```python
from build123d import *
from build123d.topology import SkipClean

# Parameters (mm, degrees)
SKETCH1_R                            = 30
BOSS_EXTRUDE1_DEPTH                  = 4
BOSS_EXTRUDE2_REACH                  = 44.615
BOSS_EXTRUDE2_END_RADIUS             = 30
BOSS_EXTRUDE2_DIRECTION_2_REACH      = 44.615
BOSS_EXTRUDE2_DIRECTION_2_END_RADIUS = 30
SKETCH3_OUTSIDE_W                    = 78.092
SKETCH3_OUTSIDE_H                    = 69.092
SKETCH3_OUTSIDE_R                    = 21.5
CUT_EXTRUDE2_DEPTH                   = 12.5
BOSS_EXTRUDE3_DEPTH                  = 18
BOSS_EXTRUDE4_DEPTH                  = 15
BOSS_EXTRUDE5_DEPTH                  = 15
CUT_EXTRUDE3_DEPTH                   = 44.292609069
CUT_EXTRUDE3_DEPTH_BACK              = 44.292609069
SKETCH8_R                            = 2
CUT_EXTRUDE8_DEPTH                   = 48.077064479
CUT_EXTRUDE8_DEPTH_BACK              = 48.077064479
CUT_EXTRUDE9_DEPTH                   = 59.659818207
CUT_EXTRUDE11_DEPTH                  = 20
CUT_EXTRUDE12_DEPTH                  = 20
CUT_EXTRUDE13_DEPTH                  = 20
CUT_EXTRUDE14_DEPTH                  = 44.292609069
CUT_EXTRUDE14_DEPTH_BACK             = 44.292609069
SKETCH25_W                           = 66.075437062
SKETCH25_H                           = 20.142243048
SKETCH26_R                           = 5
CUT_EXTRUDE15_DEPTH                  = 24
SKETCH27_R                           = 1.5
CUT_EXTRUDE16_DEPTH                  = 30
SKETCH28_R                           = 5
CUT_EXTRUDE17_DEPTH                  = 3
CUT_EXTRUDE18_DEPTH                  = 43.690748412
CUT_EXTRUDE18_DEPTH_BACK             = 43.690748412
SKETCH29_W                           = 43.412566799
SKETCH29_H                           = 13.326200919
SKETCH32_W                           = 50
SKETCH32_H                           = 12
BOSS_EXTRUDE6_DEPTH                  = 18
SKETCH35_W                           = 14
SKETCH35_H                           = 15
BOSS_EXTRUDE7_DEPTH                  = 9
CUT_EXTRUDE19_DEPTH                  = 49.746794766
CUT_EXTRUDE19_DEPTH_BACK             = 49.746794766
SKETCH37_R                           = 2
SKETCH36_R                           = 2
CUT_EXTRUDE20_DEPTH                  = 15
SKETCH39_W                           = 14
SKETCH39_H                           = 15
BOSS_EXTRUDE8_DEPTH                  = 9
SKETCH40_R                           = 2
CUT_EXTRUDE21_DEPTH                  = 10
CUT_EXTRUDE22_START                  = -9
SKETCH41_R                           = 5
CUT_EXTRUDE22_DEPTH                  = 9
CUT_EXTRUDE23_START                  = -9
SKETCH42_R                           = 5
CUT_EXTRUDE23_DEPTH                  = 9
FILLET1_R                            = 3
CUT_EXTRUDE24_START                  = -19
CUT_EXTRUDE24_OUTLINE_R              = 1.5
CUT_EXTRUDE24_DEPTH                  = 19
CUT_EXTRUDE24_START_2                = -7
CUT_EXTRUDE24_2_DEPTH                = 14


with BuildPart() as part:
    # Sketch1 → Boss-Extrude1 (new body)
    with BuildSketch(Plane(origin=(0, 0, 0), x_dir=(1, 0, 0), z_dir=(0, 1, 0))):
        with Locations(Location((0, 0, 0), (0, 0, 270))):
            Circle(SKETCH1_R)
    extrude(amount=BOSS_EXTRUDE1_DEPTH)

    # Boss-Extrude2: up to this cylinder (the profile starts inside it)
    with SkipClean():  # the faces are left unmerged after this step: merging them gives an invalid solid
        boss_extrude2_end = Plane(origin=(0, 9.396175, 0), z_dir=(0, -1, 0)) * Cylinder(BOSS_EXTRUDE2_END_RADIUS, 150.23, mode=Mode.PRIVATE)
        # Sketch2 → Boss-Extrude2 (add, up to the surface)
        with BuildSketch(Plane(origin=(0, 0, 0), x_dir=(0, 0, -1), z_dir=(1, 0, 0)), mode=Mode.PRIVATE) as boss_extrude2_sk1:
            Polygon((0, 4), (21.5, 4), (9, 16.5), (-9, 16.5), (-21.5, 4), align=None)
        boss_extrude2_tool1 = extrude(boss_extrude2_sk1.sketch, amount=BOSS_EXTRUDE2_REACH, mode=Mode.PRIVATE) & boss_extrude2_end
        add(boss_extrude2_tool1.solids().sort_by_distance((0, 9.396175, 0))[0])

    # Boss-Extrude2 direction 2: up to this cylinder (the profile starts inside it)
    with SkipClean():  # the faces are left unmerged after this step: merging them gives an invalid solid
        boss_extrude2_direction_2_end = Plane(origin=(0, 9.396175, 0), z_dir=(0, -1, 0)) * Cylinder(BOSS_EXTRUDE2_DIRECTION_2_END_RADIUS, 150.23, mode=Mode.PRIVATE)
        # Sketch2 → Boss-Extrude2 direction 2 (add, up to the surface)
        with BuildSketch(Plane(origin=(0, 0, 0), x_dir=(0, 0, -1), z_dir=(1, 0, 0)), mode=Mode.PRIVATE) as boss_extrude2_direction_2_sk1:
            Polygon((0, 4), (21.5, 4), (9, 16.5), (-9, 16.5), (-21.5, 4), align=None)
        boss_extrude2_direction_2_tool1 = extrude(boss_extrude2_direction_2_sk1.sketch, amount=-BOSS_EXTRUDE2_DIRECTION_2_REACH, mode=Mode.PRIVATE) & boss_extrude2_direction_2_end
        add(boss_extrude2_direction_2_tool1.solids().sort_by_distance((0, 9.396175, 0))[0])

    # SurfaceCut1
    split(bisect_by=Plane(origin=(0, 12.75, -12.75), x_dir=(1, 0, 0), z_dir=(0, 0.7071067811865558, -0.7071067811865392)), keep=Keep.BOTTOM)

    # SurfaceCut2
    split(bisect_by=Plane(origin=(0, 12.75, 12.75), x_dir=(1, 0, 0), z_dir=(0, 0.7071067811865509, 0.7071067811865442)), keep=Keep.BOTTOM)

    # Sketch3 outside → Cut-Extrude2 (cut)
    with BuildSketch(Plane(origin=(0, 4, 0), x_dir=(1, 0, 0), z_dir=(0, 1, 0))):
        Rectangle(SKETCH3_OUTSIDE_W, SKETCH3_OUTSIDE_H)
        Circle(SKETCH3_OUTSIDE_R, mode=Mode.SUBTRACT)
    extrude(amount=CUT_EXTRUDE2_DEPTH, mode=Mode.SUBTRACT)

    # Sketch5 → Boss-Extrude3 (add)
    with BuildSketch(Plane(origin=(0, 0, 0), x_dir=(-1, 0, 0), z_dir=(0, -1, 0))):
        Polygon((0, -6), (-17.5, -6), (-17.5, 6), (17.5, 6), (17.5, -6), align=None)
    extrude(amount=BOSS_EXTRUDE3_DEPTH)

    # Sketch6 → Boss-Extrude4 (add)
    with BuildSketch(Plane.XZ):
        Polygon((0, 15), (7, 15), (7, 6), (-7, 6), (-7, 15), align=None)
    extrude(amount=BOSS_EXTRUDE4_DEPTH)

    # Sketch7 → Boss-Extrude5 (add)
    with BuildSketch(Plane.XZ):
        Polygon((0, -15), (7, -15), (7, -6), (-7, -6), (-7, -15), align=None)
    extrude(amount=BOSS_EXTRUDE5_DEPTH)

    # Sketch8 → Cut-Extrude3 (cut, two sides: drawn at the far end of the back side and taken through both)
    with BuildSketch(Plane.XY.offset(-CUT_EXTRUDE3_DEPTH_BACK)):
        with Locations((-12.5, -12.5)):
            Circle(SKETCH8_R)
        with Locations((12.5, -12.5)):
            Circle(SKETCH8_R)
    extrude(amount=CUT_EXTRUDE3_DEPTH + CUT_EXTRUDE3_DEPTH_BACK, mode=Mode.SUBTRACT)

    # Sketch16 → Cut-Extrude8 (cut, two sides: drawn at the far end of the back side and taken through both)
    with BuildSketch(Plane.XY.offset(6).offset(-CUT_EXTRUDE8_DEPTH_BACK)):
        Polygon((17.5, -18), (17.5, -14.5), (14, -18), align=None)
        Polygon((-17.5, -18), (-14, -18), (-17.5, -14.5), align=None)
    extrude(amount=CUT_EXTRUDE8_DEPTH + CUT_EXTRUDE8_DEPTH_BACK, mode=Mode.SUBTRACT)

    # Sketch17 → Cut-Extrude9 (cut, through all)
    with BuildSketch(Plane(origin=(10.365975269, -9.674910251, -8.062425209), x_dir=(-0.3613483622370374, 0.337258471421235, -0.8693009171531012), z_dir=(0.6355070151731325, -0.5931398808282571, -0.49428323402354774))):
        Polygon((-2.372510104, -6.189601271), (7.980636686, -0.706686759), (7.980636686, -10.965829024), align=None)
    extrude(amount=CUT_EXTRUDE9_DEPTH, mode=Mode.SUBTRACT)

    # Sketch19 → Cut-Extrude11 (cut)
    with BuildSketch(Plane(origin=(-10.365975269, -9.674910251, -8.062425209), x_dir=(0.3613483622370374, 0.33725847142123494, -0.8693009171531012), z_dir=(0.6355070151731324, 0.5931398808282571, 0.4942832340235476))):
        Polygon((-2.372510104, -6.189601271), (7.980636686, -10.965829024), (7.980636686, -0.706686759), align=None)
    extrude(amount=-CUT_EXTRUDE11_DEPTH, mode=Mode.SUBTRACT)

    # Sketch20 → Cut-Extrude12 (cut)
    with BuildSketch(Plane(origin=(-10.365975269, -9.674910251, 8.062425209), x_dir=(-0.3613483622370374, -0.3372584714212349, -0.8693009171531013), z_dir=(0.6355070151731326, 0.593139880828257, -0.49428323402354757))):
        Polygon((2.372510104, -6.189601271), (-7.980636686, -0.706686759), (-7.980636686, -10.965829024), align=None)
    extrude(amount=-CUT_EXTRUDE12_DEPTH, mode=Mode.SUBTRACT)

    # Sketch21 → Cut-Extrude13 (cut)
    with BuildSketch(Plane(origin=(10.365975269, -9.674910251, 8.062425209), x_dir=(-0.3613483622370374, 0.3372584714212349, 0.8693009171531013), z_dir=(-0.6355070151731326, 0.593139880828257, -0.49428323402354757))):
        Polygon((-2.372510104, -6.189601271), (7.980636686, -0.706686759), (7.980636686, -10.965829024), align=None)
    extrude(amount=-CUT_EXTRUDE13_DEPTH, mode=Mode.SUBTRACT)

    # Sketch25 → Cut-Extrude14 (cut, two sides: drawn at the far end of the back side and taken through both)
    with BuildSketch(Plane.XY.offset(-CUT_EXTRUDE14_DEPTH_BACK)):
        with Locations((0, -10.071121524)):
            Rectangle(SKETCH25_W, SKETCH25_H)
    extrude(amount=CUT_EXTRUDE14_DEPTH + CUT_EXTRUDE14_DEPTH_BACK, mode=Mode.SUBTRACT)

    # Sketch26 → Cut-Extrude15 (cut)
    with BuildSketch(Plane(origin=(0, 16.5, 0), x_dir=(1, 0, 0), z_dir=(0, 1, 0))):
        with Locations(Location((-8, 0, 0), (0, 0, 270))):
            Circle(SKETCH26_R)
        with Locations(Location((8, 0, 0), (0, 0, 270))):
            Circle(SKETCH26_R)
    extrude(amount=-CUT_EXTRUDE15_DEPTH, mode=Mode.SUBTRACT)

    # Sketch27 → Cut-Extrude16 (cut)
    with BuildSketch(Plane(origin=(0, 16.5, 0), x_dir=(1, 0, 0), z_dir=(0, 1, 0))):
        with Locations(Location((0, 0, 0), (0, 0, 270))):
            Circle(SKETCH27_R)
    extrude(amount=-CUT_EXTRUDE16_DEPTH, mode=Mode.SUBTRACT)

    # Sketch28 → Cut-Extrude17 (cut)
    with BuildSketch(Plane.XZ):
        with Locations(Location((0, -15, 0), (0, 0, 270))):
            Circle(SKETCH28_R)
        with Locations(Location((22, 0, 0), (0, 0, 270))):
            Circle(SKETCH28_R)
        with Locations(Location((0, 15, 0), (0, 0, 270))):
            Circle(SKETCH28_R)
        with Locations(Location((-22, 0, 0), (0, 0, 270))):
            Circle(SKETCH28_R)
        with Locations(Location((-14, 12, 0), (0, 0, 270))):
            Circle(SKETCH28_R)
        with Locations(Location((14, 12, 0), (0, 0, 270))):
            Circle(SKETCH28_R)
        with Locations(Location((14, -12, 0), (0, 0, 270))):
            Circle(SKETCH28_R)
        with Locations(Location((-14, -12, 0), (0, 0, 270))):
            Circle(SKETCH28_R)
    extrude(amount=-CUT_EXTRUDE17_DEPTH, mode=Mode.SUBTRACT)

    # Sketch29 → Cut-Extrude18 (cut, two sides: drawn at the far end of the back side and taken through both)
    with BuildSketch(Plane(origin=(0, 0, 0), x_dir=(0, 0, -1), z_dir=(1, 0, 0)).offset(-CUT_EXTRUDE18_DEPTH_BACK)):
        with Locations((0.2062834, 10.66310046)):
            Rectangle(SKETCH29_W, SKETCH29_H)
    extrude(amount=CUT_EXTRUDE18_DEPTH + CUT_EXTRUDE18_DEPTH_BACK, mode=Mode.SUBTRACT)

    # Sketch32 → Boss-Extrude6 (add)
    with BuildSketch(Plane(origin=(0, 4, 0), x_dir=(1, 0, 0), z_dir=(0, 1, 0))):
        Rectangle(SKETCH32_W, SKETCH32_H)
    extrude(amount=BOSS_EXTRUDE6_DEPTH)

    # Sketch35 → Boss-Extrude7 (add)
    with BuildSketch(Plane(origin=(0, 0, -6), x_dir=(-1, 0, 0), z_dir=(0, 0, -1))):
        with Locations((0, 11.5)):
            Rectangle(SKETCH35_W, SKETCH35_H)
    extrude(amount=BOSS_EXTRUDE7_DEPTH)

    # Sketch37 → Cut-Extrude19 (cut, two sides: drawn at the far end of the back side and taken through both)
    with BuildSketch(Plane(origin=(0, 0, -6), x_dir=(-1, 0, 0), z_dir=(0, 0, -1)).offset(-CUT_EXTRUDE19_DEPTH_BACK)):
        with Locations((-12.5, 16.5)):
            Circle(SKETCH37_R)
        with Locations((12.5, 16.5)):
            Circle(SKETCH37_R)
    extrude(amount=CUT_EXTRUDE19_DEPTH + CUT_EXTRUDE19_DEPTH_BACK, mode=Mode.SUBTRACT)

    # Sketch36 → Cut-Extrude20 (cut)
    with BuildSketch(Plane(origin=(0, 19, 0), x_dir=(1, 0, 0), z_dir=(0, 1, 0))):
        with Locations(Location((0, 10, 0), (0, 0, 270))):
            Circle(SKETCH36_R)
    extrude(amount=-CUT_EXTRUDE20_DEPTH, mode=Mode.SUBTRACT)

    # Sketch39 → Boss-Extrude8 (add)
    with BuildSketch(Plane.XY.offset(6)):
        with Locations((0, 11.5)):
            Rectangle(SKETCH39_W, SKETCH39_H)
    extrude(amount=BOSS_EXTRUDE8_DEPTH)

    # Sketch40 → Cut-Extrude21 (cut)
    with BuildSketch(Plane(origin=(0, 19, 0), x_dir=(1, 0, 0), z_dir=(0, 1, 0))):
        with Locations(Location((0, -10, 0), (0, 0, 270))):
            Circle(SKETCH40_R)
    extrude(amount=-CUT_EXTRUDE21_DEPTH, mode=Mode.SUBTRACT)

    # Sketch41 → Cut-Extrude22 (cut)
    with BuildSketch(Plane.XZ.offset(-4).offset(CUT_EXTRUDE22_START)):
        with Locations(Location((-8, 0, 0), (0, 0, 90))):
            Circle(SKETCH41_R)
    extrude(amount=CUT_EXTRUDE22_DEPTH, mode=Mode.SUBTRACT)

    # Sketch42 → Cut-Extrude23 (cut)
    with BuildSketch(Plane.XZ.offset(-4).offset(CUT_EXTRUDE23_START)):
        with Locations(Location((8, 0, 0), (0, 0, 90))):
            Circle(SKETCH42_R)
    extrude(amount=CUT_EXTRUDE23_DEPTH, mode=Mode.SUBTRACT)

    # Fillet1
    fillet1_edges = [part.edges().sort_by_distance(p)[0] for p in [
        (25, 22, 0),
    ]]
    fillet(fillet1_edges, radius=FILLET1_R)

    # Cut-Extrude24: read off the stored shape, not the designer's step
    # Cut-Extrude24 outline → Cut-Extrude24 (cut)
    with BuildSketch(Plane.XZ.offset(-4).offset(CUT_EXTRUDE24_START)):
        Circle(CUT_EXTRUDE24_OUTLINE_R)
    extrude(amount=CUT_EXTRUDE24_DEPTH, mode=Mode.SUBTRACT)

    # Cut-Extrude24 2 outline → Cut-Extrude24 2 (cut)
    with BuildSketch(Plane.XY.offset(CUT_EXTRUDE24_START_2)):
        with BuildLine():
            Line((-25, 22), (-25, 19))
            ThreePointArc((-25, 19), (-24.121320344, 21.121320344), (-22, 22))
            Line((-22, 22), (-25, 22))
        make_face()
    extrude(amount=CUT_EXTRUDE24_2_DEPTH, mode=Mode.SUBTRACT)


solid = part.part
```
CAD build for the part. Positions are in the model's coordinates, mm. A direction names the side the tool comes from. Coordinates: 2 decimals unless noted, no trailing zeros. Order: outer loops, then holes, each group sorted by start corner. A loop starts at its lowest first (then second) coordinate and runs counter-clockwise, first axis right, second up.
(1) Saw through at B-B, the plane y = 1.5. Count the separate pieces of the cut face and the enclosed holes in it, and give its area (3 significant figures).
Solution:
separate pieces: 1
enclosed holes: 11
area: 1,740 mm2
(2) Which spindle directions (+Z, -Z, +X, -X, +Y, -Y) get a long thin tool onto all of the face, cutting with end or side? Do faces 5 (the face through (-2, 19, 11)), 6 (the face through (14, 3, -12)), 7 (the face through (0, 4, -10)), 8 (the face through (7, 11, -10)). Say none if no direction does.
Solution:
face 5: +Z, +X, -X, +Y
face 6: -Y
face 7: +Y
face 8: -Z, +X, +Y
(3) Pin check, flat tips, straight feed: pin 1 Ø7 at (x, y) = (0.5, 11.5) entering from -Z; pin 2 Ø1 at (x, y) = (17.5, 4) entering from +Z; pin 3 Ø2 at (y, z) = (12, -0.5) entering from -X. Stop position of each tip, or through.
Solution:
pin 1: stops at z = -15
pin 2: stops at z = 22
pin 3: stops at x = -25
(4) Saw through at A-A, the plane y = 16.5. Write the cut outline in (x, z), and give its area (3 significant figures).
Solution:
outline: (-25, -6) - (-14.5, -6) - (-14.5, 6) - (-25, 6) - close; (-10.5, -6) - (-7, -6) - (-7, -15) - (7, -15) - (7, -6) - (10.5, -6) - (10.5, 6) - (7, 6) - (7, 15) - (-7, 15) - (-7, 6) - (-10.5, 6) - close; (14.5, -6) - (25, -6) - (25, 6) - (14.5, 6) - close; hole circle Ø4 at (0, -10); hole circle Ø4 at (0, 10); hole circle Ø3 at (0, 0)
area: 724 mm2
(5) Drill centre lines: L1, parallel to X at y = 17.25, z = 1; L2, parallel to Z at x = 1, y = 11.75; L3, parallel to X at y = 1.2, z = -15. Where is each one in solid material? Low to high.
Solution:
L1: x = -25 to -14.35, -10.65 to -1.12, 1.12 to 10.65, 14.35 to 25
L2: z = -15 to -11.73, -8.27 to -1.12, 1.12 to 8.27, 11.73 to 15
L3: x = -25.98 to -18, -10 to -5, 5 to 10, 18 to 25.98
(6) Mould opens along Z. For faces 1 (the face through (-7, 11, 10)), 2 (the face through (-14, 3, -12)), 3 (the face through (9.564, 1.479, 9.693)), 4 (the face through (0, 12, -15)) say: released by +Z, released by -Z, zero draft, split by the parting line, or undercut.
Solution:
face 1: zero draft
face 2: undercut
face 3: undercut
face 4: released by -Z
(7) Saw through at D-D, the plane x = 4. Write the cut outline in (y, z), and give its area (3 significant figures).
Solution:
outline: (0, -25.5) - (4, -21.5) - (4, -15) - (19, -15) - (19, -6) - (22, -6) - (22, 6) - (19, 6) - (19, 15) - (4, 15) - (4, 21.5) - (0, 25.5) - (0, 18) - (3, 18) - (3, 12) - (0, 12) - (0, 3) - (13, 3) - (13, -3) - (0, -3) - (0, -12) - (3, -12) - (3, -18) - (0, -18) - close
area: 560 mm2
(8) Saw through at C-C, the plane y = 11.75. Write the cut outline in (x, z).
Solution:
outline: (-25, -6) - (-7, -6) - (-7, -15) - (7, -15) - (7, -6) - (25, -6) - (25, 6) - (7, 6) - (7, 15) - (-7, 15) - (-7, 6) - (-25, 6) - close; hole circle Ø10 at (-8, 0); hole circle Ø4 at (0, -10); hole circle Ø4 at (0, 10); hole circle Ø3 at (0, 0); hole circle Ø10 at (8, 0)
